The listing builds one solid part. Answer for the finished solid, in the listing's coordinates (mm). Face numbers are marked on the shaded views. Round coordinates to 2 decimals unless told otherwise and drop trailing zeros. Write each loop counter-clockwise with the first axis right and the second up, starting at its lowest first coordinate (ties: lowest second). Pieces come first, ordered by that corner, then holes. Notation, with made-up numbers: (-30, 9.5) - (2, 9.5) arc R28 ccw to (2, 32.5) - close; hole circle Ø9 at (-8.75, 74.25). An arc over 180 degrees is marked (long way). Use a Markdown table: item, result. Add a question column.
1) Determine the mould class of the marked faces 1 and 2 for opening direction X: +X half, -X half, draft (parallel to the pull), parting line (faces both ways), or undercut.
2) A cutting plane is placed at A-A (z = -28.5). Give the vertices of the cut face in (x, y).
3) A cutting plane is placed at C-C (x = 61.5). Give the vertices of the cut face in (y, z).
4) Each of these flat-tipped pins is pushed along its axis until it touches: P1, Ø3, axis at x = 98, z = 0, coming from the -Y side; P2, Ø1.2, axis at x = 45, z = -88, coming from the -Y side. Where does it stop, or does it pass through?
5) Find the intervals of material crossed by probe 1 along X at (y, z) = (6.75, -11); probe 2 along X at (y, z) = (5.45, 0); probe 3 along Z at (x, y) = (-47, 6.75), in increasing order. Write a range as from..to.
6) A cutting plane is placed at B-B (x = -59.5). Give the vertices of the cut face in (y, z).
```python
from build123d import *

# Parameters (mm, degrees)
SKETCH1_W           = 210
SKETCH1_H           = 190
SKETCH1_W_2         = 206
SKETCH1_H_2         = 186
BOSS_EXTRUDE1_DEPTH = 5
SKETCH7_R           = 1
CUT_EXTRUDE1_DEPTH  = 2
SKETCH8_R           = 1
CUT_EXTRUDE2_DEPTH  = 2
CUT_EXTRUDE3_START  = -2
SKETCH6_R           = 1
CUT_EXTRUDE3_DEPTH  = 2
CUT_EXTRUDE4_START  = -2
SKETCH5_R           = 1
CUT_EXTRUDE4_DEPTH  = 2
SKETCH9_W           = 210
SKETCH9_H           = 190
SKETCH9_R           = 1
SKETCH9_W_2         = 96
SKETCH9_H_2         = 166
SKETCH9_W_3         = 82
SKETCH9_H_3         = 13
BOSS_EXTRUDE3_DEPTH = 2


with BuildPart() as part:
    # Sketch1 → Boss-Extrude1 (new body)
    with BuildSketch(Plane(origin=(0, 0, 0), x_dir=(1, 0, 0), z_dir=(0, 1, 0))):
        Rectangle(SKETCH1_W, SKETCH1_H)
        Rectangle(SKETCH1_W_2, SKETCH1_H_2, mode=Mode.SUBTRACT)
    extrude(amount=BOSS_EXTRUDE1_DEPTH)

    # Sketch7 → Cut-Extrude1 (cut)
    with BuildSketch(Plane(origin=(105, 0, 0), x_dir=(0, 0, -1), z_dir=(1, 0, 0))):
        with Locations((0, 3)):
            Circle(SKETCH7_R)
    extrude(amount=-CUT_EXTRUDE1_DEPTH, mode=Mode.SUBTRACT)

    # Sketch8 → Cut-Extrude2 (cut)
    with BuildSketch(Plane.XY.offset(95)):
        with Locations((0, 3)):
            Circle(SKETCH8_R)
    extrude(amount=-CUT_EXTRUDE2_DEPTH, mode=Mode.SUBTRACT)

    # Sketch6 → Cut-Extrude3 (cut)
    with BuildSketch(Plane(origin=(0, 0, -95), x_dir=(-1, 0, 0), z_dir=(0, 0, -1)).offset(CUT_EXTRUDE3_START)):
        with Locations(Location((0, 3, 0), (0, 0, 180))):
            Circle(SKETCH6_R)
    extrude(amount=CUT_EXTRUDE3_DEPTH, mode=Mode.SUBTRACT)

    # Sketch5 → Cut-Extrude4 (cut)
    with BuildSketch(Plane.ZY.offset(105).offset(CUT_EXTRUDE4_START)):
        with Locations(Location((0, 3, 0), (0, 0, 180))):
            Circle(SKETCH5_R)
    extrude(amount=CUT_EXTRUDE4_DEPTH, mode=Mode.SUBTRACT)

    # Sketch9 → Boss-Extrude3 (add)
    with BuildSketch(Plane(origin=(0, 5, 0), x_dir=(1, 0, 0), z_dir=(0, 1, 0))):
        Rectangle(SKETCH9_W, SKETCH9_H)
        with Locations(Location((98, 0, 0), (0, 0, 270))):
            Circle(SKETCH9_R, mode=Mode.SUBTRACT)
        with Locations(Location((45, 88, 0), (0, 0, 270))):
            Circle(SKETCH9_R, mode=Mode.SUBTRACT)
        with Locations(Location((-8, 0, 0), (0, 0, 270))):
            Circle(SKETCH9_R, mode=Mode.SUBTRACT)
        with Locations(Location((45, -88, 0), (0, 0, 270))):
            Circle(SKETCH9_R, mode=Mode.SUBTRACT)
        with Locations((45, 0)):
            Rectangle(SKETCH9_W_2, SKETCH9_H_2, mode=Mode.SUBTRACT)
        with Locations((-54, -40.5)):
            Rectangle(SKETCH9_W_3, SKETCH9_H_3, mode=Mode.SUBTRACT)
        with Locations((-54, -12.5)):
            Rectangle(SKETCH9_W_3, SKETCH9_H_3, mode=Mode.SUBTRACT)
        with Locations((-54, 16.5)):
            Rectangle(SKETCH9_W_3, SKETCH9_H_3, mode=Mode.SUBTRACT)
        with Locations((-54, 42.5)):
            Rectangle(SKETCH9_W_3, SKETCH9_H_3, mode=Mode.SUBTRACT)
        with Locations((-54, 66.5)):
            Rectangle(SKETCH9_W_3, SKETCH9_H_3, mode=Mode.SUBTRACT)
    extrude(amount=BOSS_EXTRUDE3_DEPTH)


solid = part.part
```
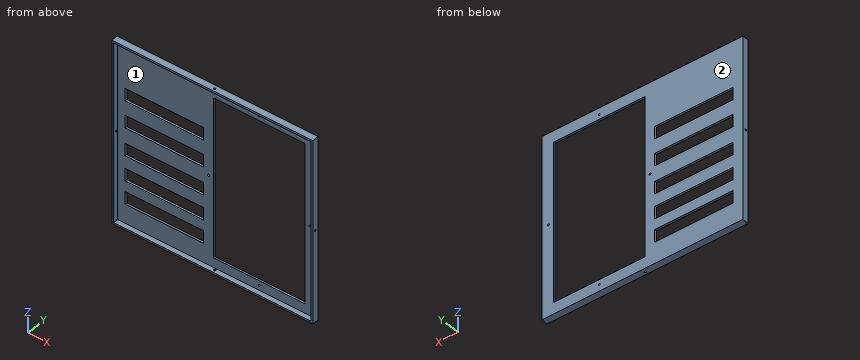
Entries:
| question | item | result |
|---|---|---|
| 1 | face 1 | undercut |
| 1 | face 2 | draft |
| 2 | outline | (-105, 0) - (-103, 0) - (-103, 5) - (-3, 5) - (-3, 7) - (-105, 7) - close; (93, 5) - (103, 5) - (103, 0) - (105, 0) - (105, 7) - (93, 7) - close |
| 3 | outline | (0, -95) - (7, -95) - (7, -83) - (5, -83) - (5, -93) - (0, -93) - close; (0, 93) - (5, 93) - (5, 83) - (7, 83) - (7, 95) - (0, 95) - close |
| 4 | P1 | stops at y = 5 |
| 4 | P2 | passes through |
| 5 | probe 1 | x = -105..-95, -13..-3, 93..105 |
| 5 | probe 2 | x = -105..-9, -7..-3, 93..97, 99..105 |
| 5 | probe 3 | z = -95..-73, -60..-49, -36..-23, -10..6, 19..34, 47..95 |
| 6 | outline | (0, -95) - (7, -95) - (7, -73) - (5, -73) - (5, -93) - (0, -93) - close; (0, 93) - (5, 93) - (5, 47) - (7, 47) - (7, 95) - (0, 95) - close; (5, -60) - (7, -60) - (7, -49) - (5, -49) - close; (5, -36) - (7, -36) - (7, -23) - (5, -23) - close; (5, -10) - (7, -10) - (7, 6) - (5, 6) - close; (5, 19) - (7, 19) - (7, 34) - (5, 34) - close |
